CAD build for the part. Positions are in the model's coordinates, mm. A direction names the side the tool comes from. Coordinates: 2 decimals unless noted, no trailing zeros. Write each loop counter-clockwise with the first axis right and the second up, starting at its lowest first coordinate (ties: lowest second). Pieces come first, ordered by that corner, then holes. Notation, with made-up numbers: (-11.75, -23.75) - (1.25, -23.75) arc R21 ccw to (1.25, -10.75) - close; hole circle Ø8 at (78, 26). An arc over 180 degrees is marked (long way). Answer in a Markdown table with one row per item. Add a question column.
Q1. Band-saw the part on C-C (y = 4.5). List the corners of the cut face in (x, z), and give its area (3 significant figures).
Q2. Band-saw the part on B-B (z = -7). List the corners of the cut face in (x, y), and give its area (3 significant figures).
Q3. Band-saw the part on D-D (x = 8.5). List the corners of the cut face in (y, z), and give its area (3 significant figures).
Q4. Two-plate mould, pull along Z, no slides. Class faces 1 (the flat face through (-22.97, -0.07, 10.85)), 2 (the cylindrical face through (-42.7, 0.07, -12.87)), 3 (the cylindrical face through (-42.546, -0.07, 6.169)): +Z half, -Z half, draft (parallel to the pull), parting line (faces both ways), or undercut.
Q5. 3-axis set-ups, long thin cutter, end or side, ignore diameter. For faces 4 (the flat face through (3, 0, -10.158)), 5 (the flat face through (9, 0, -5.158)), 6 (the flat face through (-23, 0, -10.158)): which of +Z, -Z, +X, -X, +Y, -Y reach the whole face in a straight line?
Q6. Drill centre lines: line 1 along X through (y, z) = (-1.75, -11.75); line 2 along Z through (x, y) = (-10, 0); line 3 along X through (y, z) = (4, -7.75). Where is each one in solid material? Low to high. Write a range as from..to.
Q7. Pin check, flat tips, straight feed: pin 1 (3 mm diameter, centred on x = 3, y = -3, fed in from +Z); pin 2 (3 mm diameter, centred on y = -1, z = -2, fed in from -X); pin 3 (4 mm diameter, centred on x = 1.5, y = 2, fed in from +Z); pin 4 (8 mm diameter, centred on x = -21, z = -5, fed in from +Y). Stop position of each tip, or through.
Q8. Band-saw the part on A-A (x = -28). List the corners of the cut face in (y, z), and give its area (3 significant figures).
```python
from build123d import *

# Parameters (mm, degrees)
PAD_DEPTH    = 5
FILLET_R     = 3
CHAMFER_SIZE = 2
FILLET001_R  = 1


with BuildPart() as part:
    # Sketch → Pad (new body, symmetric)
    with BuildSketch(Plane.XZ):
        Polygon((-43.099497, 8.82665), (0, 13.158312), (0, -10.158312), (5, -10.158312), (6.819851, -5.158312), (10.819851, -5.158312), (10.819851, -13.158312), (0, -13.158312), (-43, -13.158312), (-43, -10.158312), (-3, -10.158312), (-3, 9.841688), (-42.799497, 5.841688), align=None)
    extrude(amount=PAD_DEPTH, both=True)

    # Fillet
    fillet_edges = [part.edges().sort_by_distance(p)[0] for p in [
        (0, 0, 13.158312),
    ]]
    fillet(fillet_edges, radius=FILLET_R)

    # Chamfer
    chamfer_edges = [part.edges().sort_by_distance(p)[0] for p in [
        (0, 0, -10.158312),
    ]]
    chamfer(chamfer_edges, length=CHAMFER_SIZE)

    # Fillet001
    fillet001_edges = [part.edges().sort_by_distance(p)[0] for p in [
        (-42.799497, 0, 5.841688),
        (-43.099497, 0, 8.82665),
        (-43, 0, -10.158312),
        (-43, 0, -13.158312),
        (10.819851, 0, -5.158312),
        (6.819851, 0, -5.158312),
        (10.819851, 0, -13.158312),
    ]]
    fillet(fillet001_edges, radius=FILLET001_R)


solid = part.part
```
Checked values:
| question | item | result |
|---|---|---|
| 1 | outline | (-43, -12.16) arc R1 ccw to (-42, -13.16) - (9.82, -13.16) arc R1 ccw to (10.82, -12.16) - (10.82, -6.16) arc R1 ccw to (9.82, -5.16) - (7.52, -5.16) arc R1 ccw to (6.58, -5.82) - (5, -10.16) - (2, -10.16) - (0, -8.16) - (0, 9.84) arc R3 ccw to (-3.3, 12.83) - (-42.1, 8.93) arc R1 ccw to (-43, 7.83) - (-42.9, 6.84) arc R1 ccw to (-41.8, 5.94) - (-3, 9.84) - (-3, -10.16) - (-42, -10.16) arc R1 ccw to (-43, -11.16) - close |
| 1 | area | 374 mm² |
| 2 | outline | (-3, -5) - (0, -5) - (0, 5) - (-3, 5) - close; (6.15, -5) - (10.82, -5) - (10.82, 5) - (6.15, 5) - close |
| 2 | area | 76.7 mm² |
| 3 | outline | (-5, -13.16) - (5, -13.16) - (5, -5.16) - (-5, -5.16) - close |
| 3 | area | 80.0 mm² |
| 4 | face 1 | +Z half |
| 4 | face 2 | -Z half |
| 4 | face 3 | undercut |
| 5 | face 4 | +Z, +Y, -Y |
| 5 | face 5 | +Z, +X, +Y, -Y |
| 5 | face 6 | -X, +Y, -Y |
| 6 | line 1 | x = -43..10.82 |
| 6 | line 2 | z = -13.16..-10.16, 9.14..12.15 |
| 6 | line 3 | x = -3..0, 5.88..10.82 |
| 7 | pin 1 | stops at z = -9.66 |
| 7 | pin 2 | stops at x = -3 |
| 7 | pin 3 | stops at z = 11.5 |
| 7 | pin 4 | passes through |
| 8 | outline | (-5, -13.16) - (5, -13.16) - (5, -10.16) - (-5, -10.16) - close; (-5, 7.33) - (5, 7.33) - (5, 10.34) - (-5, 10.34) - close |
| 8 | area | 60.2 mm² |
